Can you work these out from the model? Positions are in its coordinate system, mm. Face numbers are marked on the shaded views. A direction names the side the tool comes from. Coordinates: 2 decimals unless noted, no trailing zeros. Order: outer loops, then holes, each group sorted by start corner. A loop starts at its lowest first (then second) coordinate and runs counter-clockwise, first axis right, second up. Notation, with made-up numbers: (-29, 38.5) -> (18, 38.5) arc R12 ccw to (18, 55.5) -> close; hole circle Ø8 at (82.5, 77). An arc over 180 degrees is marked (long way). Answer in a Markdown table with one row per item. Add a question column.
1. We'd pull the mould along X, two halves only. Please class the marked faces 1, 2 and 3: pulls with the +X half, pulls with the -X half, needs draft (parallel to the pull), parting line crosses it, or undercut.
2. On a 3-axis mill with a long thin cutter (end or side, diameter ignored), from which of +Z, -Z, +X, -X, +Y, -Y can I reach the whole of each face in a straight line? I mean the marked faces 4 and 5. Say none if no direction works.
3. Imagine slicing it at A-A on z = 1.5. Write out the boundary of the cut face in (x, y) (3 decimals), plus the area to 3 significant figures.
4. Will this pin go through, and if not, where does the flat tip stop? pin 1 (4.5 mm diameter, centred on x = -2.5, y = 6.5, fed in from +Z).
5. Imagine slicing it at C-C on y = 5.5. Write out the boundary of the cut face in (x, z) (3 decimals).
6. If I drill on line 1 along X through (y, z) = (7.5, 2.5) (3 decimals); line 2 along X through (y, z) = (4.5, 4.75); line 3 along Z through (x, y) = (0.5, 6.5), over which ranges is the centre line in solid material (lowest first)? Write a range as [from, to].
7. Imagine slicing it at B-B on x = 3.5. Write out the boundary of the cut face in (y, z).
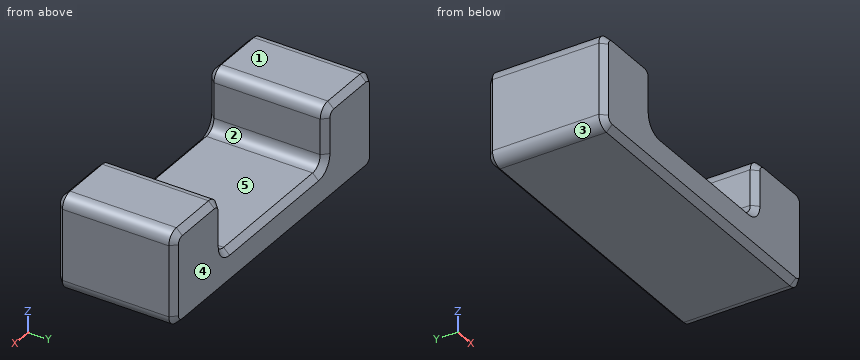
from build123d import *

# Parameters (mm, degrees)
BOSS_EXTRUDE1_DEPTH = 10
FILLET1_R           = 1
CHAMFER1_SIZE       = 0.5


with BuildPart() as part:
    # Sketch1 → Boss-Extrude1 (new body)
    with BuildSketch(Plane(origin=(0, 0, 0), x_dir=(1, 0, 0), z_dir=(0, 1, 0))):
        Polygon((-13.125, 0), (-13.125, -5), (-6.875, -5), (-6.875, 0), (6.875, 0), (6.875, -5), (13.125, -5), (13.125, 0), (13.125, 3), (-13.125, 3), align=None)
    extrude(amount=BOSS_EXTRUDE1_DEPTH)

    # Fillet1
    fillet1_edges = [part.edges().sort_by_distance(p)[0] for p in [
        (-6.875, 5, 0),
        (-6.875, 5, 5),
        (-13.125, 5, 5),
        (-13.125, 5, -3),
        (13.125, 5, -3),
        (13.125, 5, 5),
        (6.875, 5, 5),
        (6.875, 5, 0),
    ]]
    fillet(fillet1_edges, radius=FILLET1_R)

    # Chamfer1
    chamfer1_edges = [part.edges().sort_by_distance(p)[0] for p in [
        (0, 0, -3),
        (0, 10, -3),
        (0, 0, 0),
        (-6.875, 0, 2.5),
        (-10, 0, 5),
        (-13.125, 0, 1),
        (13.125, 0, 1),
        (10, 0, 5),
        (6.875, 0, 2.5),
        (-12.832106781, 0, 4.707106781),
        (-7.167893219, 0, 4.707106781),
        (-12.832106781, 0, -2.707106781),
        (7.167893219, 0, 4.707106781),
        (12.832106781, 0, 4.707106781),
        (12.832106781, 0, -2.707106781),
        (13.125, 10, 1),
        (0, 10, 0),
        (6.875, 10, 2.5),
        (10, 10, 5),
        (-13.125, 10, 1),
        (-10, 10, 5),
        (-6.875, 10, 2.5),
        (-12.832106781, 10, 4.707106781),
        (-7.167893219, 10, 4.707106781),
        (-12.832106781, 10, -2.707106781),
        (7.167893219, 10, 4.707106781),
        (12.832106781, 10, 4.707106781),
        (12.832106781, 10, -2.707106781),
        (6.582106781, 0, 0.292893219),
        (6.582106781, 10, 0.292893219),
        (-6.582106781, 0, 0.292893219),
        (-6.582106781, 10, 0.292893219),
    ]]
    chamfer(chamfer1_edges, length=CHAMFER1_SIZE)


solid = part.part
Answers follow:
| question | item | result |
|---|---|---|
| 1 | face 1 | needs draft |
| 1 | face 2 | undercut |
| 1 | face 3 | pulls with the -X half |
| 2 | face 4 | +Z, -Z, +X, -X, +Y |
| 2 | face 5 | +Z, +Y, -Y |
| 3 | outline | (-13.125, 0.5) -> (-12.625, 0) -> (-7.375, 0) -> (-6.875, 0.5) -> (-6.875, 9.5) -> (-7.375, 10) -> (-12.625, 10) -> (-13.125, 9.5) -> close; (6.875, 0.5) -> (7.375, 0) -> (12.625, 0) -> (13.125, 0.5) -> (13.125, 9.5) -> (12.625, 10) -> (7.375, 10) -> (6.875, 9.5) -> close |
| 3 | area | 124 mm² |
| 4 | pin 1 | stops at z = 0 |
| 5 | outline | (-13.125, -2) arc R1 ccw to (-12.125, -3) -> (12.125, -3) arc R1 ccw to (13.125, -2) -> (13.125, 4) arc R1 ccw to (12.125, 5) -> (7.875, 5) arc R1 ccw to (6.875, 4) -> (6.875, 1) arc R1 cw to (5.875, 0) -> (-5.875, 0) arc R1 cw to (-6.875, 1) -> (-6.875, 4) arc R1 ccw to (-7.875, 5) -> (-12.125, 5) arc R1 ccw to (-13.125, 4) -> close |
| 6 | line 1 | x = [-13.125, -6.875], [6.875, 13.125] |
| 6 | line 2 | x = [-12.79, -7.21], [7.21, 12.79] |
| 6 | line 3 | z = [-3, 0] |
| 7 | outline | (0, -2.5) -> (0.5, -3) -> (9.5, -3) -> (10, -2.5) -> (10, -0.5) -> (9.5, 0) -> (0.5, 0) -> (0, -0.5) -> close |
